from build123d import *

# Parameters (mm, degrees)
SKETCH3_W           = 254
SKETCH3_H           = 82.55
BOSS_EXTRUDE2_DEPTH = 6.35
SKETCH4_W           = 6.35
SKETCH4_H           = 12.7
SKETCH4_W_2         = 12.7
SKETCH4_H_2         = 6.35
CUT_EXTRUDE2_DEPTH  = 6.35


with BuildPart() as part:
    # Sketch3 → Boss-Extrude2 (new body)
    with BuildSketch(Plane(origin=(0, 0, 0), x_dir=(-1, 0, 0), z_dir=(0, 1, 0))):
        with Locations((127, 41.275)):
            Rectangle(SKETCH3_W, SKETCH3_H)
    extrude(amount=BOSS_EXTRUDE2_DEPTH)

    # Sketch4 → Cut-Extrude2 (cut)
    with BuildSketch(Plane(origin=(0, 6.35, 0), x_dir=(-1, 0, 0), z_dir=(0, 1, 0))):
        with Locations((3.175, 25.4)):
            Rectangle(SKETCH4_W, SKETCH4_H)
        with Locations((3.175, 50.8)):
            Rectangle(SKETCH4_W, SKETCH4_H)
        with Locations((250.825, 25.4)):
            Rectangle(SKETCH4_W, SKETCH4_H)
        with Locations((250.825, 50.8)):
            Rectangle(SKETCH4_W, SKETCH4_H)
        with Locations((50.8, 3.175)):
            Rectangle(SKETCH4_W_2, SKETCH4_H_2)
        with Locations((25.4, 3.175)):
            Rectangle(SKETCH4_W_2, SKETCH4_H_2)
        with Locations((76.2, 3.175)):
            Rectangle(SKETCH4_W_2, SKETCH4_H_2)
        with Locations((101.6, 3.175)):
            Rectangle(SKETCH4_W_2, SKETCH4_H_2)
        with Locations((127, 3.175)):
            Rectangle(SKETCH4_W_2, SKETCH4_H_2)
        with Locations((177.8, 3.175)):
            Rectangle(SKETCH4_W_2, SKETCH4_H_2)
        with Locations((152.4, 3.175)):
            Rectangle(SKETCH4_W_2, SKETCH4_H_2)
        with Locations((203.2, 3.175)):
            Rectangle(SKETCH4_W_2, SKETCH4_H_2)
        with Locations((228.6, 3.175)):
            Rectangle(SKETCH4_W_2, SKETCH4_H_2)
    extrude(amount=-CUT_EXTRUDE2_DEPTH, mode=Mode.SUBTRACT)


solid = part.part
Here's how the part is built. I have some questions about the finished solid (model axes, mm). A direction names the side the tool comes from. Round coordinates to 2 decimals unless told otherwise and drop trailing zeros. Order: outer loops, then holes, each group sorted by start corner. A loop starts at its lowest first (then second) coordinate and runs counter-clockwise, first axis right, second up. Notation, with made-up numbers: (-20.5, 63.5) -> (1.5, 63.5) arc R25 cw to (1.5, 89.5) -> close; hole circle Ø4 at (-26, 34.25). An arc over 180 degrees is marked (long way). Return JSON: item names as keys, results as strings.
Q1. If we mould it in two halves opening along Z, with no side actions, what happens to faces 1 (the flat face through (-196.85, 3, 3)), 2 (the flat face through (-6.35, 3, 25)), 3 (the flat face through (-6.35, 3, 51)), 4 (the flat face through (-244, 3, 0))? For each: released by +Z, released by -Z, zero draft, split by the parting line, or undercut.
Filled sheet:
{"face 1": "zero draft", "face 2": "undercut", "face 3": "undercut", "face 4": "released by -Z"}
Q2. I need wall thicknesses on line 1 along Z through (x, y) = (-56, 6); line 2 along X through (y, z) = (2.5, 56.5). Which ranges of each line are inside material? Lowest first, please. Write a range as from..to.
Filled sheet:
{"line 1": "z = 6.35..82.55", "line 2": "x = -247.65..-6.35"}
Q3. If we section it at A-A on z = 52: List the corners of the cut face in (x, y) for me, plus the area to 3 significant figures.
Filled sheet:
{"outline": "(-247.65, 0) -> (-6.35, 0) -> (-6.35, 6.35) -> (-247.65, 6.35) -> close", "area": "1,530 mm^2"}
Q4. If we section it at B-B on x = -102: List the corners of the cut face in (y, z) for me.
Filled sheet:
{"outline": "(0, 6.35) -> (6.35, 6.35) -> (6.35, 82.55) -> (0, 82.55) -> close"}
Q5. For pin 1 Ø3 at (x, y) = (-203.5, 2) entering from -Z, with a flat end and sliding along its axis, tell me the tip position at first contact or that it passes through.
Filled sheet:
{"pin 1": "stops at z = 6.35"}
Q6. Which directions (+Z, -Z, +X, -X, +Y, -Y) give clear straight access to the entire face, cutting with the end or side of a thin tool? Please do faces 5 (the flat face through (-31.75, 3, 3)), 6 (the flat face through (-3, 3, 31.75)), 7 (the flat face through (-140, 3, 0)).
Filled sheet:
{"face 5": "-Z, +Y, -Y", "face 6": "+X, +Y, -Y", "face 7": "-Z, +X, -X, +Y, -Y"}
